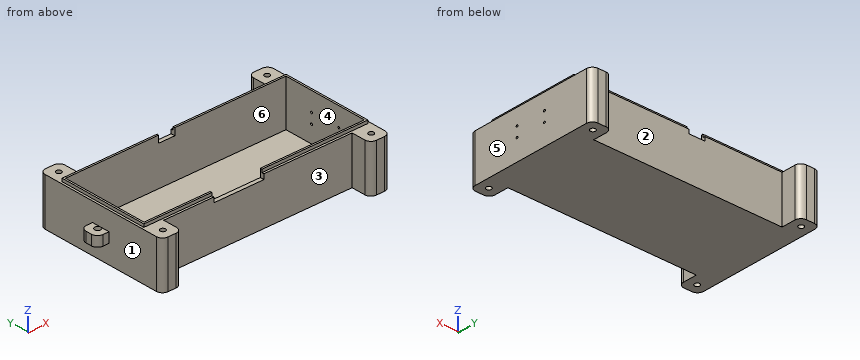
```python
from build123d import *

# Parameters (mm, degrees)
SKETCH_W        = 114
SKETCH_H        = 47
PAD_DEPTH       = 25
THICKNESS_T     = -2
SKETCH001_W     = 114
SKETCH001_H     = 1.1
POCKET_DEPTH    = 1.5
SKETCH002_W     = 1.1
SKETCH002_H     = 47
POCKET001_DEPTH = 1.5
SKETCH003_W     = 10
SKETCH003_H     = 23.5
PAD001_DEPTH    = 10
SKETCH004_W     = 10
SKETCH004_H     = 23.5
PAD002_DEPTH    = 10
SKETCH005_R     = 1.3
POCKET002_DEPTH = 23.5
SKETCH006_R     = 0.5
POCKET003_DEPTH = 2
SKETCH007_W     = 9
SKETCH007_H     = 5
PAD003_DEPTH    = 6
SKETCH009_R     = 1.5
POCKET004_DEPTH = 5
FILLET_R        = 3
FILLET001_R     = 3
FILLET002_R     = 3
SKETCH010_W     = 25
SKETCH010_H     = 4
POCKET005_DEPTH = 2
SKETCH011_W     = 8
SKETCH011_H     = 3.5
POCKET006_DEPTH = 2


with BuildPart() as part:
    # Sketch → Pad (new body)
    with BuildSketch(Plane.XY):
        Rectangle(SKETCH_W, SKETCH_H)
    extrude(amount=PAD_DEPTH)

    # Thickness
    thickness_openings = [part.faces().sort_by_distance(p)[0] for p in [
        (0, 0, 25),
    ]]
    offset(amount=THICKNESS_T, openings=thickness_openings)

    # Sketch001 (on Face6 of Thickness) → Pocket (cut)
    with BuildSketch(Plane.XY.offset(25)):
        with Locations((0, -22.95)):
            Rectangle(SKETCH001_W, SKETCH001_H)
        with Locations((0, 22.95)):
            Rectangle(SKETCH001_W, SKETCH001_H)
    extrude(amount=-POCKET_DEPTH, mode=Mode.SUBTRACT)

    # Sketch002 (on Face6 of Pocket) → Pocket001 (cut)
    with BuildSketch(Plane.XY.offset(25)):
        with Locations((56.45, 0)):
            Rectangle(SKETCH002_W, SKETCH002_H)
        with Locations((-56.45, 0)):
            Rectangle(SKETCH002_W, SKETCH002_H)
    extrude(amount=-POCKET001_DEPTH, mode=Mode.SUBTRACT)

    # Sketch003 (on Face4 of Pocket001) → Pad001 (join)
    with BuildSketch(Plane(origin=(0, 23.5, 0), x_dir=(-1, 0, 0), z_dir=(0, 1, 0))):
        with Locations((-52, 11.75)):
            Rectangle(SKETCH003_W, SKETCH003_H)
        with Locations((52, 11.75)):
            Rectangle(SKETCH003_W, SKETCH003_H)
    extrude(amount=PAD001_DEPTH)

    # Sketch004 (on Face1 of Pad001) → Pad002 (join)
    with BuildSketch(Plane.XZ.offset(23.5)):
        with Locations((-52, 11.75)):
            Rectangle(SKETCH004_W, SKETCH004_H)
        with Locations((52, 11.75)):
            Rectangle(SKETCH004_W, SKETCH004_H)
    extrude(amount=PAD002_DEPTH)

    # Sketch005 (on Face12 of Pad002) → Pocket002 (cut)
    with BuildSketch(Plane.XY.offset(23.5)):
        with Locations((-52, 28.5)):
            Circle(SKETCH005_R)
        with Locations((52, 28.5)):
            Circle(SKETCH005_R)
        with Locations((52, -28.5)):
            Circle(SKETCH005_R)
        with Locations((-52, -28.5)):
            Circle(SKETCH005_R)
    extrude(amount=-POCKET002_DEPTH, mode=Mode.SUBTRACT)

    # Sketch006 (on Face12 of Pocket002) → Pocket003 (cut)
    with BuildSketch(Plane.YZ.offset(57)):
        with Locations((7.5, 10.5)):
            Circle(SKETCH006_R)
        with Locations((7.5, 15.5)):
            Circle(SKETCH006_R)
        with Locations((-7.5, 10.5)):
            Circle(SKETCH006_R)
        with Locations((-7.5, 15.5)):
            Circle(SKETCH006_R)
    extrude(amount=-POCKET003_DEPTH, mode=Mode.SUBTRACT)

    # Sketch007 (on Face4 of Pocket003) → Pad003 (join)
    with BuildSketch(Plane(origin=(-57, 0, 0), x_dir=(0, -1, 0), z_dir=(-1, 0, 0))):
        with Locations((0, 11.75)):
            Rectangle(SKETCH007_W, SKETCH007_H)
    extrude(amount=PAD003_DEPTH)

    # Sketch009 (on Face22 of Pad003) → Pocket004 (cut)
    with BuildSketch(Plane.XY.offset(14.25)):
        with Locations((-58.5, 0)):
            Circle(SKETCH009_R)
    extrude(amount=-POCKET004_DEPTH, mode=Mode.SUBTRACT)

    # Fillet
    fillet_edges = [part.edges().sort_by_distance(p)[0] for p in [
        (-57, -33.5, 11.75),
        (-47, -33.5, 11.75),
        (47, -33.5, 11.75),
        (57, -33.5, 11.75),
    ]]
    fillet(fillet_edges, radius=FILLET_R)

    # Fillet001
    fillet001_edges = [part.edges().sort_by_distance(p)[0] for p in [
        (-63, -4.5, 11.75),
        (-63, 4.5, 11.75),
    ]]
    fillet(fillet001_edges, radius=FILLET001_R)

    # Fillet002
    fillet002_edges = [part.edges().sort_by_distance(p)[0] for p in [
        (57, 33.5, 11.75),
        (47, 33.5, 11.75),
        (-47, 33.5, 11.75),
        (-57, 33.5, 11.75),
    ]]
    fillet(fillet002_edges, radius=FILLET002_R)

    # Sketch010 (on Face17 of Fillet002) → Pocket005 (cut)
    with BuildSketch(Plane.XZ.offset(23.5)):
        with Locations((-9.5, 23)):
            Rectangle(SKETCH010_W, SKETCH010_H)
    extrude(amount=-POCKET005_DEPTH, mode=Mode.SUBTRACT)

    # Sketch011 (on Face13 of Pocket005) → Pocket006 (cut)
    with BuildSketch(Plane(origin=(0, 23.5, 0), x_dir=(-1, 0, 0), z_dir=(0, 1, 0))):
        with Locations((4.5, 23.25)):
            Rectangle(SKETCH011_W, SKETCH011_H)
    extrude(amount=-POCKET006_DEPTH, mode=Mode.SUBTRACT)


solid = part.part
```
Work out the finished part from the listing and answer in its coordinate system (mm). Face numbers are marked on the shaded views. A direction names the side the tool comes from. Give positions to 0.01 mm unless a question says otherwise; leave off trailing zeros. Loops run counter-clockwise (first coordinate to the right, second up) from the corner with the lowest first, then second, coordinate; pieces in that order, holes last. Notation, with made-up numbers: (-14, 58) -> (12, 58) arc R8 ccw to (12, 63) -> close; hole circle Ø7 at (-29, -16). An arc over 180 degrees is marked (long way). One line per question, with ' | ' between items. Start each with the question number.
1) Section C-C, the plane x = 52 is taken. Determine the outline of the cut face in (y, z).
2) Section A-A, the plane x = -58.5 is taken. Determine the outline of the cut face in (y, z).
3) Section B-B, the plane z = 6.25 is taken. Determine the outline of the cut face in (x, y), then the cut area to 3 significant figures.
4) Straight lines are drawn through the part: L1, parallel to Y at x = -52, z = 10.5; L2, parallel to Z at x = 56.4, y = 7.5; L3, parallel to Y at x = -13, z = 2.75. For each, find the intervals that lie inside material, in ascending order.
5) Each of these flat-tipped pins is pushed along its axis until it touches: pin 1 (2 mm diameter, centred on x = -52, y = 28.5, fed in from +Z); pin 2 (0.9 mm diameter, centred on x = -58.5, z = 12, fed in from -Y); pin 3 (0.9 mm diameter, centred on x = -59, z = 12.5, fed in from +Y); pin 4 (1.5 mm diameter, centred on y = -17.5, z = 9, fed in from -X). Where does it stop, or does it pass through?
6) Section D-D, the plane y = -28.5 is taken. Determine the outline of the cut face in (x, z).
7) Determine the mould class of the marked faces 1, 2, 3 and 4 for opening direction Y: +Y half, -Y half, draft (parallel to the pull), parting line (faces both ways), or undercut.
8) For the marked faces 5 and 6, determine the directions among +Z, -Z, +X, -X, +Y, -Y from which every point of the face is accessible in a straight line to the end or side of a thin tool.
Resolved:
1) outline: (-33.5, 0) -> (-29.8, 0) -> (-29.8, 23.5) -> (-33.5, 23.5) -> close; (-27.2, 0) -> (27.2, 0) -> (27.2, 23.5) -> (22.4, 23.5) -> (22.4, 25) -> (21.5, 25) -> (21.5, 2) -> (-21.5, 2) -> (-21.5, 25) -> (-22.4, 25) -> (-22.4, 23.5) -> (-27.2, 23.5) -> close; (29.8, 0) -> (33.5, 0) -> (33.5, 23.5) -> (29.8, 23.5) -> close
2) outline: (-4.5, 9.25) -> (-1.5, 9.25) -> (-1.5, 14.25) -> (-4.5, 14.25) -> close; (1.5, 9.25) -> (4.5, 9.25) -> (4.5, 14.25) -> (1.5, 14.25) -> close
3) outline: (-57, -30.5) arc R3 ccw to (-54, -33.5) -> (-50, -33.5) arc R3 ccw to (-47, -30.5) -> (-47, -23.5) -> (47, -23.5) -> (47, -30.5) arc R3 ccw to (50, -33.5) -> (54, -33.5) arc R3 ccw to (57, -30.5) -> (57, 30.5) arc R3 ccw to (54, 33.5) -> (50, 33.5) arc R3 ccw to (47, 30.5) -> (47, 23.5) -> (-47, 23.5) -> (-47, 30.5) arc R3 ccw to (-50, 33.5) -> (-54, 33.5) arc R3 ccw to (-57, 30.5) -> close; hole (-55, -21.5) -> (55, -21.5) -> (55, 21.5) -> (-55, 21.5) -> close; hole circle Ø2.6 at (-52, -28.5); hole circle Ø2.6 at (-52, 28.5); hole circle Ø2.6 at (52, -28.5); hole circle Ø2.6 at (52, 28.5) | area: 991 mm2
4) L1: -33.5 to -29.8, -27.2 to -21.5, 21.5 to 27.2, 29.8 to 33.5 | L2: 0 to 10, 11 to 15, 16 to 23.5 | L3: -23.5 to -21.5, 21.5 to 23.5
5) pin 1: through | pin 2: y = -4.5 | pin 3: y = 4.5 | pin 4: x = -57
6) outline: (-57, 0) -> (-53.3, 0) -> (-53.3, 23.5) -> (-57, 23.5) -> close; (-50.7, 0) -> (-47, 0) -> (-47, 23.5) -> (-50.7, 23.5) -> close; (47, 0) -> (50.7, 0) -> (50.7, 23.5) -> (47, 23.5) -> close; (53.3, 0) -> (57, 0) -> (57, 23.5) -> (53.3, 23.5) -> close
7) face 1: draft | face 2: +Y half | face 3: -Y half | face 4: undercut
8) face 5: +Z, -Z, +X, +Y, -Y | face 6: +Z
